The drawing under review shows one solid part. Ordinate dimensions are in mm from its lowest x, y, z. Coordinates: 2 decimals unless noted, no trailing zeros. Order: outer loops, then holes, each group sorted by start corner. A loop starts at its lowest first (then second) coordinate and runs counter-clockwise, first axis right, second up.
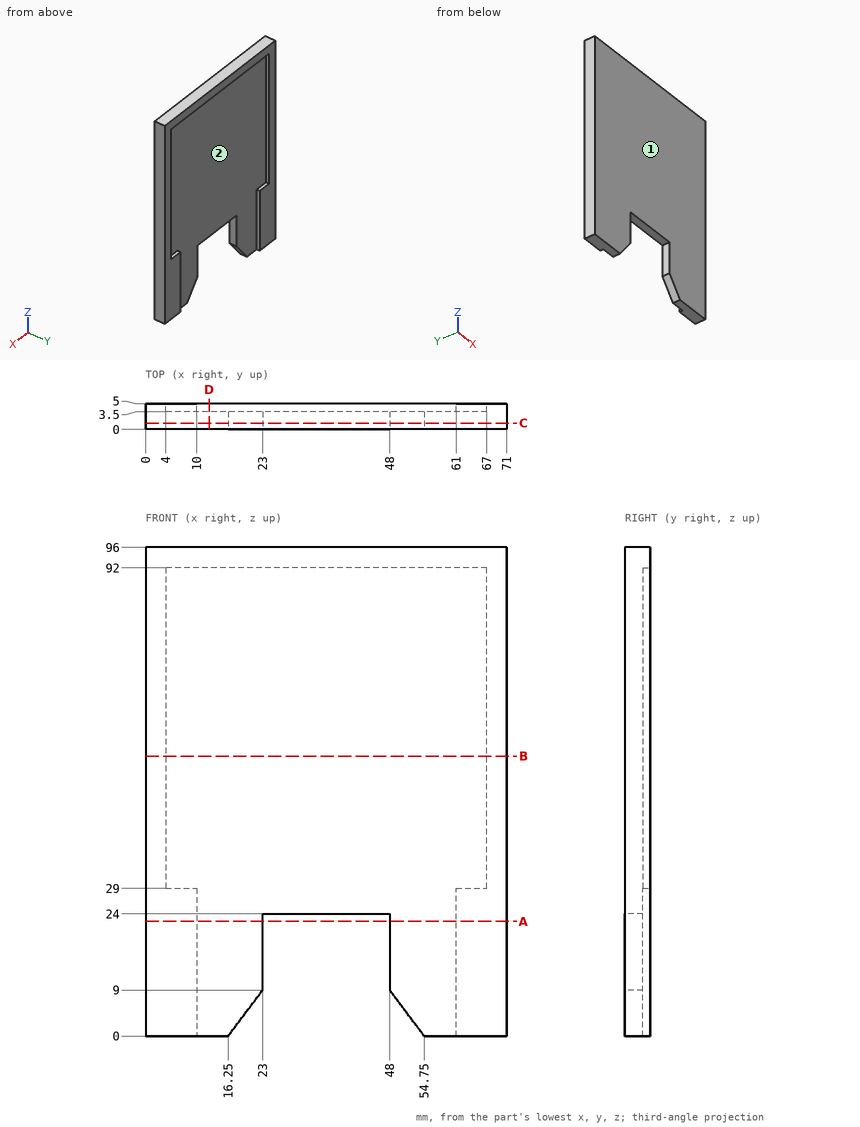
(1) Wall thickness on probe 1 along X at (y, z) = (4.65, 28); probe 2 along X at (y, z) = (3.6, 53); probe 3 along Z at (x, y) = (63.5, 4.05): over which ranges is each line inside the solid? List them lowest first.
A:
probe 1: x = 0 to 10, 61 to 71
probe 2: x = 0 to 4, 67 to 71
probe 3: z = 0 to 29, 92 to 96
(2) For pin 1 Ø1 at (x, z) = (39.5, 69) entering from +Y; pin 2 Ø1.8 at (x, y) = (32, 2.5) entering from -Z, all flat-tipped, find the tip position at first contact; note any pin that passes through.
A:
pin 1: stops at y = 3.5
pin 2: stops at z = 24
(3) We need section C-C, the plane y = 1.25. Write out the cut boundary in (x, z), and give its area (3 significant figures).
A:
outline: (0, 0) - (16.25, 0) - (23, 9) - (23, 24) - (48, 24) - (48, 9) - (54.75, 0) - (71, 0) - (71, 96) - (0, 96) - close
area: 6,160 mm2
(4) We need section A-A, the plane z = 22.5. Write out the cut boundary in (x, y), and give its area (3 significant figures).
A:
outline: (0, 0) - (23, 0) - (23, 3.5) - (10, 3.5) - (10, 5) - (0, 5) - close; (48, 0) - (71, 0) - (71, 5) - (61, 5) - (61, 3.5) - (48, 3.5) - close
area: 191 mm2
(5) Draft analysis for pull direction Z (two halves, no side actions). For the marked faces 1 and 2, state which applies: released by +Z, released by -Z, zero draft, split by the parting line, or undercut.
A:
face 1: zero draft
face 2: undercut
(6) We need section D-D, the plane x = 12.5. Write out the cut boundary in (y, z), and give its area (3 significant figures).
A:
outline: (0, 0) - (3.5, 0) - (3.5, 92) - (5, 92) - (5, 96) - (0, 96) - close
area: 342 mm2
(7) We need section B-B, the plane z = 55. Write out the cut boundary in (x, y), and give its area (4 significant figures).
A:
outline: (0, 0) - (71, 0) - (71, 5) - (67, 5) - (67, 3.5) - (4, 3.5) - (4, 5) - (0, 5) - close
area: 260.5 mm2
